```python
from build123d import *

# Parameters (mm, degrees)
SKETCH2_R           = 3.025
SKETCH2_R_2         = 1.525
BOSS_EXTRUDE2_DEPTH = 15


with BuildPart() as part:
    # Sketch2 → Boss-Extrude2 (new body)
    with BuildSketch(Plane(origin=(0, 0, 0), x_dir=(0, 0, -1), z_dir=(1, 0, 0))):
        Polygon((-56.025707453, -71.794871795), (17.987179487, -71.794871795), (17.987179487, 68.205128205), (-18.512820513, 68.205128205), align=None)
        with Locations((11.487179487, 58.205128205)):
            Circle(SKETCH2_R, mode=Mode.SUBTRACT)
        with Locations((11.487179487, 43.205128205)):
            Circle(SKETCH2_R, mode=Mode.SUBTRACT)
        with Locations((11.487179487, 28.205128205)):
            Circle(SKETCH2_R, mode=Mode.SUBTRACT)
        with Locations((11.487179487, 13.205128205)):
            Circle(SKETCH2_R, mode=Mode.SUBTRACT)
        with Locations((11.487179487, -1.794871795)):
            Circle(SKETCH2_R, mode=Mode.SUBTRACT)
        with Locations((11.487179487, -16.794871795)):
            Circle(SKETCH2_R, mode=Mode.SUBTRACT)
        with Locations((11.487179487, -31.794871795)):
            Circle(SKETCH2_R, mode=Mode.SUBTRACT)
        with Locations((11.487179487, -46.794871795)):
            Circle(SKETCH2_R, mode=Mode.SUBTRACT)
        with Locations((0.987179487, 48.205128205)):
            Circle(SKETCH2_R_2, mode=Mode.SUBTRACT)
        with Locations((-12.012820513, 48.205128205)):
            Circle(SKETCH2_R_2, mode=Mode.SUBTRACT)
        with Locations((0.987179487, 33.205128205)):
            Circle(SKETCH2_R_2, mode=Mode.SUBTRACT)
        with Locations((-12.012820513, 33.205128205)):
            Circle(SKETCH2_R_2, mode=Mode.SUBTRACT)
        with Locations((0.987179487, 18.205128205)):
            Circle(SKETCH2_R_2, mode=Mode.SUBTRACT)
        with Locations((-12.012820513, 18.205128205)):
            Circle(SKETCH2_R_2, mode=Mode.SUBTRACT)
        with Locations((0.987179487, 3.205128205)):
            Circle(SKETCH2_R_2, mode=Mode.SUBTRACT)
        with Locations((-12.012820513, 3.205128205)):
            Circle(SKETCH2_R_2, mode=Mode.SUBTRACT)
        with Locations((0.987179487, -11.794871795)):
            Circle(SKETCH2_R_2, mode=Mode.SUBTRACT)
        with Locations((-12.012820513, -11.794871795)):
            Circle(SKETCH2_R_2, mode=Mode.SUBTRACT)
        with Locations((0.987179487, -26.794871795)):
            Circle(SKETCH2_R_2, mode=Mode.SUBTRACT)
        with Locations((-12.012820513, -26.794871795)):
            Circle(SKETCH2_R_2, mode=Mode.SUBTRACT)
        with Locations((0.987179487, -41.794871795)):
            Circle(SKETCH2_R_2, mode=Mode.SUBTRACT)
        with Locations((-12.012820513, -41.794871795)):
            Circle(SKETCH2_R_2, mode=Mode.SUBTRACT)
        with Locations((0.987179487, -56.794871795)):
            Circle(SKETCH2_R_2, mode=Mode.SUBTRACT)
        with Locations((-12.012820513, -56.794871795)):
            Circle(SKETCH2_R_2, mode=Mode.SUBTRACT)
    extrude(amount=BOSS_EXTRUDE2_DEPTH)


solid = part.part
```
Model file for the job. Use its own axes, mm. Coordinates: 2 decimals unless noted, no trailing zeros. Order: outer loops, then holes, each group sorted by start corner. A loop starts at its lowest first (then second) coordinate and runs counter-clockwise, first axis right, second up. Notation, with made-up numbers: (87, -20) -> (120, -20) arc R16 ccw to (120, -14) -> close; hole circle Ø2 at (-28, 18). An arc over 180 degrees is marked (long way). Answer as a JSON object with one key per item and string values. Group by question number.
1) Flat gauge pins, fed straight in: pin 1 (2.5 mm diameter, centred on y = -56.79, z = -0.99, fed in from -X); pin 2 (4 mm diameter, centred on y = -26.79, z = 12.01, fed in from +X); pin 3 (6 mm diameter, centred on x = 12.5, y = 39.5, fed in from +Z); pin 4 (2 mm diameter, centred on x = 12.5, y = -41.5, fed in from +Z). Where does each tip first touch, or does it go through?
2) Drill centre lines: L1, parallel to Z at x = 2.5, y = -27.5; L2, parallel to Z at x = 13.25, y = -55.5; L3, parallel to Z at x = 1.5, y = 29. Where is each one in solid material? Low to high.
3) Cut at C-C, the plane y = 6.5. Write the cut outline in (x, z).
4) Pull direction Z, two halves, no side cores. Call faces 1 (the face through (7.395, 49.717, -0.789)), 2 (the face through (7, -3, -17.987)), 3 (the face through (7, 68.205, 0)): +Z half, -Z half, draft (parallel to the pull), parting line (faces both ways), or undercut.
5) Cut at A-A, the plane x = 7.75. Count the separate pieces of the cut face and the enclosed holes in it, then the cut area to 3 significant figures.
6) Cut at D-D, the plane z = 27. Write the cut outline in (x, y).
Check values:
{
 "1": {"pin 1": "passes through", "pin 2": "stops at x = 15", "pin 3": "stops at z = 27.01", "pin 4": "stops at z = 48.18"},
 "2": {"L1": "z = -17.99 to -2.34, 0.37 to 10.66, 13.37 to 44.16", "L2": "z = -17.99 to -1.79, -0.18 to 11.21, 12.82 to 51.66", "L3": "z = -17.99 to -14.41, -8.57 to 29.02"},
 "3": {"outline": "(0, -17.99) -> (15, -17.99) -> (15, 35.05) -> (0, 35.05) -> close"},
 "4": {"face 1": "undercut", "face 2": "-Z half", "face 3": "draft"},
 "5": {"separate pieces": "1", "enclosed holes": "24", "area": "7,390 mm²"},
 "6": {"outline": "(0, -71.79) -> (15, -71.79) -> (15, 36.53) -> (0, 36.53) -> close"}
}
